Autodesk Inventor part; units mm, degrees
ref_plane "YZ Plane" through (0, 0, 0) normal (1, 0, 0) x (0, 1, 0)
ref_plane "XZ Plane" through (0, 0, 0) normal (0, 1, 0) x (-1, 0, 0)
ref_plane "XY Plane" through (0, 0, 0) normal (0, 0, 1) x (1, 0, 0)
sketch "Sketch1" plane through (0, 0, 0) normal (0, 1, 0) x (-1, 0, 0)
  circle A0 centre (0, 0) radius 31.75
  circle A1 centre (0, 0) radius 12.7
  circle A2 centre (0, 0) radius 25.4
  line L0 (24.7979, 5.4976) -> (12.399, 2.7488)
  line L1 (12.399, -2.7488) -> (24.7979, -5.4976)
  circle A3 centre (0, 0) radius 7.9375
  line L2 (0, 0) -> (7.9375, 0) construction
  line L3 (8.58, 9.3634) -> (17.16, 18.7268)
  line L4 (7.6379, 24.2244) -> (3.819, 12.1122)
  line L5 (-3.819, 12.1122) -> (-7.6379, 24.2244)
  line L6 (-17.16, 18.7268) -> (-8.58, 9.3634)
  line L7 (-12.399, 2.7488) -> (-24.7979, 5.4976)
  line L8 (-24.7979, -5.4976) -> (-12.399, -2.7488)
  line L9 (-8.58, -9.3634) -> (-17.16, -18.7268)
  line L10 (-7.6379, -24.2244) -> (-3.819, -12.1122)
  line L11 (3.819, -12.1122) -> (7.6379, -24.2244)
  line L12 (17.16, -18.7268) -> (8.58, -9.3634)
  dimension "d3" = 15.875
  dimension "d0" = 63.5
  dimension "d1" = 25.4
  dimension "d2" = 50.8
  dimension "d4" = 25
  dimension "d7" = 360
extrude "Extrusion1" add sketch "Sketch1" along normal blind 12.7 contours A0 | A1 | A1 L0 A2 L1 | A1 L4 A2 L3 | L12 A2 L11 A1 | A1 L6 A2 L5 | L10 A2 L9 A1 | A1 L8 A2 L7
fillet "Fillet1" radius 3.175 4 edges at (-3.819, 6.35, -12.1122) (3.819, 6.35, -12.1122) (7.6379, 6.35, -24.2244) (-7.6379, 6.35, -24.2244)
pattern_circular "Circular Pattern1" count 6 over 360 about axis through (0, 0, 0) along (0, 1, 0) of "Fillet1"
properties part number "2.5in flex"
For this review, take the finished solid that the model builds, in its own axes (mm). Coordinates: 2 decimals unless noted, no trailing zeros. Order: outer loops, then holes, each group sorted by start corner. A loop starts at its lowest first (then second) coordinate and runs counter-clockwise, first axis right, second up. Notation, with made-up numbers: (40, 18) -> (93, 18) arc R16 ccw to (93, 42) -> close; hole circle Ø4 at (28, 68). An arc over 180 degrees is marked (long way). Use CSV: the item, a comma, the result in double quotes. Start each with the question number.
Item 1: We need section C-C, the plane y = 5. Give the number of separate pieces and of enclosed holes in the cut face, then the cut area to 3 significant figures.
Item 2: Insertion check: pin 1 (1.5 mm diameter, centred on x = -2, y = 5.5, fed in from -Z); pin 2 (3 mm diameter, centred on y = 5.5, z = 2.5, fed in from -X); pin 3 (1 mm diameter, centred on y = 6.5, z = -7.5, fed in from -X). Each pin has a flat end and moves straight along its axis. Give the tip position at first contact, or say it passes through.
Item 3: We need section A-A, the plane x = 0. Give the boundary of the cut face in (y, z), then the cut area to 3 significant figures.
Item 4: We need section B-B, the plane z = 0. Give the boundary of the cut face in (x, y), then the cut area to 3 significant figures.
Item 5: We need section D-D, the plane z = 18.5. Give the boundary of the cut face in (x, y).
Item 6: Draft analysis for pull direction Z (two halves, no side actions). For faces 1 (the face through (17.253, 6.439, 17.247)), 2 (the face through (-13.043, 6.439, 3.644)), state which applies: pulls with the +Z half, pulls with the -Z half, needs draft (parallel to the pull), parting line crosses it, or undercut.
Item 7: Wall thickness on probe 1 along Z at (x, y) = (0, 5.25); probe 2 along Z at (x, y) = (-2.5, 11.5); probe 3 along X at (y, z) = (6, -5): over which ranges is each line inside the solid? List them lowest first.
Derived:
1,separate pieces,"1"
1,enclosed holes,"7"
1,area,"2,130 mm^2"
2,pin 1,"stops at z = -31.73"
2,pin 2,"stops at x = -31.73"
2,pin 3,"stops at x = -30.97"
3,outline,"(0, -31.75) -> (12.7, -31.75) -> (12.7, -25.4) -> (0, -25.4) -> close; (0, -12.7) -> (12.7, -12.7) -> (12.7, -7.94) -> (0, -7.94) -> close; (0, 7.94) -> (12.7, 7.94) -> (12.7, 12.7) -> (0, 12.7) -> close; (0, 25.4) -> (12.7, 25.4) -> (12.7, 31.75) -> (0, 31.75) -> close"
3,area,"282 mm^2"
4,outline,"(-31.75, 0) -> (-7.94, 0) -> (-7.94, 12.7) -> (-31.75, 12.7) -> close; (7.94, 0) -> (31.75, 0) -> (31.75, 12.7) -> (7.94, 12.7) -> close"
4,area,"605 mm^2"
5,outline,"(-25.8, 0) -> (-5.83, 0) -> (-5.83, 12.7) -> (-25.8, 12.7) -> close; (5.83, 0) -> (25.8, 0) -> (25.8, 12.7) -> (5.83, 12.7) -> close"
6,face 1,"undercut"
6,face 2,"undercut"
7,probe 1,"z = -31.75 to -25.4, -12.7 to -7.94, 7.94 to 12.7, 25.4 to 31.75"
7,probe 2,"z = -31.65 to -25.28, -12.73 to -7.53, 7.53 to 12.73, 25.28 to 31.65"
7,probe 3,"x = -31.35 to -22.17, -11.68 to -6.16, 6.16 to 11.68, 22.17 to 31.35"
